Here's the drawing with two shaded views (mm, measured from the low corner). I have some questions. A direction names the side the tool comes from. Coordinates: 2 decimals unless noted, no trailing zeros. Write each loop counter-clockwise with the first axis right and the second up, starting at its lowest first coordinate (ties: lowest second). Pieces come first, ordered by that corner, then holes.
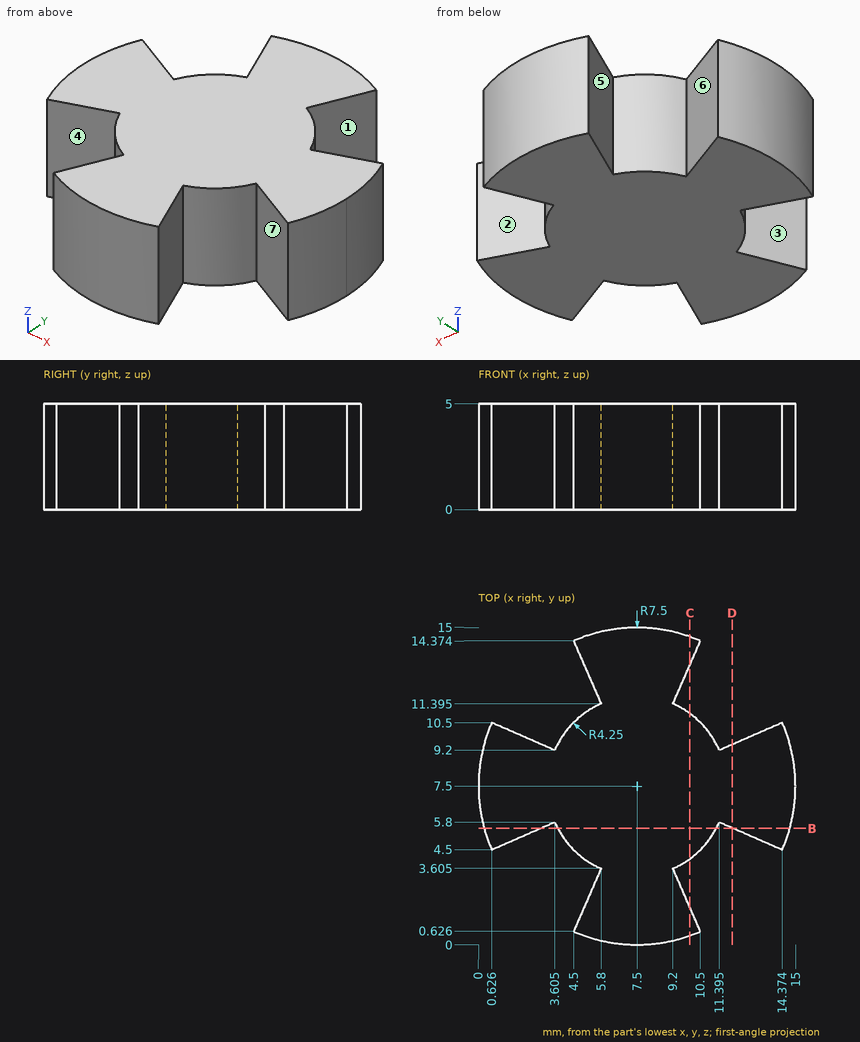
Item 1: If we mould it in two halves opening along Y, with no side actions, what happens to the marked faces 5, 6 and 7? For each: released by +Y, released by -Y, zero draft, split by the parting line, or undercut.
Item 2: I want a section at B-B, the plane y = 5.5. List the corners of the cut face in (x, z) for me.
Item 3: I want a section at D-D, the plane x = 12. List the corners of the cut face in (y, z) for me, then the cut area to 3 significant figures.
Item 4: I want a section at C-C, the plane x = 10. List the corners of the cut face in (y, z) for me, then the cut area to 3 significant figures.
Item 5: Which directions (+Z, -Z, +X, -X, +Y, -Y) give clear straight access to the entire face, cutting with the end or side of a thin tool? Please do the marked faces 1, 2, 3 and 4.
Item 6: If I drill on line 1 along Y through (x, z) = (5.25, 0.5) (1 decimal); line 2 along X through (y, z) = (5, 3.2) (1 decimal); line 3 along X through (y, z) = (14, 0.2), over which ranges is the centre line in solid material (lowest first)?
Item 7: Will these pins go through, and if not, where does the flat tip stop? pin 1 Ø2 at (y, z) = (6, 1.5) entering from -X; pin 2 Ø1.5 at (x, z) = (9, 4.5) entering from +Y.
Taken from the geometry:
1. face 5: undercut
1. face 6: released by +Y
1. face 7: released by -Y
2. outline: (0.27, 0) - (2.92, 0) - (2.92, 5) - (0.27, 5) - close; (3.75, 0) - (11.25, 0) - (11.25, 5) - (3.75, 5) - close; (12.08, 0) - (14.73, 0) - (14.73, 5) - (12.08, 5) - close
3. outline: (5.54, 0) - (9.46, 0) - (9.46, 5) - (5.54, 5) - close
3. area: 19.6 mm2
4. outline: (0.43, 0) - (1.77, 0) - (1.77, 5) - (0.43, 5) - close; (4.06, 0) - (10.94, 0) - (10.94, 5) - (4.06, 5) - close; (13.23, 0) - (14.57, 0) - (14.57, 5) - (13.23, 5) - close
4. area: 47.8 mm2
5. face 1: +Z, -Z, +X
5. face 2: +Z, -Z, +Y
5. face 3: +Z, -Z, -X
5. face 4: +Z, -Z, -Y
6. line 1: y = 0.3 to 2.3, 3.9 to 11.1, 12.7 to 14.7
6. line 2: x = 0.4 to 1.8, 4.1 to 10.9, 13.2 to 14.6
6. line 3: x = 4.66 to 10.34
7. pin 1: stops at x = 0.02
7. pin 2: stops at y = 14.96
